```python
from build123d import *
from OCP.BRepFilletAPI import BRepFilletAPI_MakeChamfer

# Parameters (mm, degrees)
SKETCH1_W           = 8
SKETCH1_H           = 19.5
BOSS_EXTRUDE1_DEPTH = 2
FILLET1_R           = 1.6
CUT_EXTRUDE1_DEPTH  = 0.1
SKETCH4_R           = 2.5
SKETCH4_R_2         = 2.25
BOSS_EXTRUDE2_DEPTH = 0.2
CHAMFER1_SIZE       = 0.15
CHAMFER1_SIZE2      = 0.08660254
SKETCH5_W           = 8
SKETCH5_H           = 0.1
CUT_EXTRUDE2_DEPTH  = 1
FILLET2_R           = 0.1


with BuildPart() as part:
    # Sketch1 → Boss-Extrude1 (new body)
    with BuildSketch(Plane.XY):
        with Locations((4, 9.75)):
            Rectangle(SKETCH1_W, SKETCH1_H)
    extrude(amount=BOSS_EXTRUDE1_DEPTH)

    # Fillet1
    fillet1_edges = [part.edges().sort_by_distance(p)[0] for p in [
        (0, 19.5, 1),
        (8, 19.5, 1),
        (8, 0, 1),
        (0, 0, 1),
    ]]
    fillet(fillet1_edges, radius=FILLET1_R)

    # Sketch3 → Cut-Extrude1 (cut)
    with BuildSketch(Plane.XY.offset(2)):
        with BuildLine():
            Line((4.35, 17.3), (4.35, 16.1))
            ThreePointArc((4.35, 16.1), (4, 15.75), (3.65, 16.1))
            Line((3.65, 16.1), (3.65, 17.3))
            ThreePointArc((3.65, 17.3), (4, 17.65), (4.35, 17.3))
        make_face()
        with BuildLine():
            ThreePointArc((2.649265581, 16.627272727), (4, 14.65), (5.350734419, 16.627272727))
            ThreePointArc((5.350734419, 16.627272727), (4.897422349, 16.826039343), (4.698655734, 16.372727273))
            ThreePointArc((4.698655734, 16.372727273), (4, 15.35), (3.301344266, 16.372727273))
            ThreePointArc((3.301344266, 16.372727273), (3.102577651, 16.826039343), (2.649265581, 16.627272727))
        make_face()
    extrude(amount=-CUT_EXTRUDE1_DEPTH, mode=Mode.SUBTRACT)

    # Sketch4 → Boss-Extrude2 (add)
    with BuildSketch(Plane.XY.offset(2)):
        with Locations(Location((4, 16.1, 0), (0, 0, 180))):
            Circle(SKETCH4_R)
        with Locations((4, 16.1)):
            Circle(SKETCH4_R_2, mode=Mode.SUBTRACT)
    extrude(amount=BOSS_EXTRUDE2_DEPTH)

    # Chamfer1: one chamfer whose edges measure the first distance from different faces: ONE call of the kernel's chamfer builder (chamfer() names one face for all edges)
    chamfer1_edges_1 = [part.edges().sort_by_distance(p)[0] for p in [
        (6.5, 16.1, 2.2),
    ]]
    chamfer1_side_1 = [part.faces().sort_by_distance(p)[0] for p in [
        (6.5, 16.1, 2.1),
    ]]
    chamfer1_edges_2 = [part.edges().sort_by_distance(p)[0] for p in [
        (1.75, 16.1, 2.2),
    ]]
    chamfer1_side_2 = [part.faces().sort_by_distance(p)[0] for p in [
        (6.429289322, 16.1, 2.2),
    ]]
    chamfer1 = BRepFilletAPI_MakeChamfer(part.part.solid().wrapped)
    for e in chamfer1_edges_1:
        chamfer1.Add(CHAMFER1_SIZE, CHAMFER1_SIZE2, e.wrapped, chamfer1_side_1[0].wrapped)  # the first distance lies on this face
    for e in chamfer1_edges_2:
        chamfer1.Add(CHAMFER1_SIZE, CHAMFER1_SIZE2, e.wrapped, chamfer1_side_2[0].wrapped)  # the first distance lies on this face
    add(Compound.cast(chamfer1.Shape()), mode=Mode.REPLACE)

    # Sketch5 → Cut-Extrude2 (cut)
    with BuildSketch(Plane.XY.offset(2)):
        with Locations((4, 12.45)):
            Rectangle(SKETCH5_W, SKETCH5_H)
    extrude(amount=-CUT_EXTRUDE2_DEPTH, mode=Mode.SUBTRACT)

    # Fillet2
    # the kernel refuses this fillet: 0.1 mm, written as the material it adds along each edge
    with BuildSketch(Plane(origin=(4, 16.1, 2), x_dir=(-1, 0, 0), z_dir=(0, 1, 0))) as fillet2_piece_1:
        with BuildLine():
            CenterArc((2.58660254, 0.1), FILLET2_R, 210, 60)
            Line((2.58660254, 0), (2.5, 0))
            Line((2.5, 0), (2.5, 0.05))
        make_face()
    revolve(axis=Axis((4, 16.1, 2), (0, 0, 1)))
    # the kernel refuses this fillet: 0.1 mm, written as the material it takes off along each edge
    with BuildSketch(Plane(origin=(8, 1.6, 2), x_dir=(0, 0, -1), z_dir=(0, 1, 0)), Plane(origin=(0, 12.65, 2), x_dir=(0, 0, -1), z_dir=(0, -1, 0))) as fillet2_2_piece_1:
        with BuildLine():
            CenterArc((FILLET2_R, FILLET2_R), FILLET2_R, 180, 90)
            Line((0, FILLET2_R), (0, 0))
            Line((0, 0), (FILLET2_R, 0))
        make_face()
    extrude(amount=11.05, mode=Mode.SUBTRACT)
    with BuildSketch(Plane(origin=(1.6, 0, 2), x_dir=(0, 1, 0), z_dir=(1, 0, 0)), Plane(origin=(6.4, 19.5, 2), x_dir=(0, -1, 0), z_dir=(-1, 0, 0))) as fillet2_2_piece_2:
        with BuildLine():
            CenterArc((FILLET2_R, -FILLET2_R), FILLET2_R, 90, 90)
            Line((0, -FILLET2_R), (0, 0))
            Line((0, 0), (FILLET2_R, 0))
        make_face()
    extrude(amount=4.8, mode=Mode.SUBTRACT)
    with BuildSketch(Plane(origin=(0, 17.9, 2), x_dir=(1, 0, 0), z_dir=(0, -1, 0)), Plane(origin=(8, 12.25, 2), x_dir=(-1, 0, 0), z_dir=(0, 1, 0))) as fillet2_2_piece_3:
        with BuildLine():
            CenterArc((FILLET2_R, -FILLET2_R), FILLET2_R, 90, 90)
            Line((0, -FILLET2_R), (0, 0))
            Line((0, 0), (FILLET2_R, 0))
        make_face()
    extrude(amount=5.65, mode=Mode.SUBTRACT)
    with BuildSketch(Plane(origin=(1.6, 17.9, 2), x_dir=(0, 1, 0), z_dir=(1, 0, 0))) as fillet2_2_piece_4:
        with BuildLine():
            CenterArc((1.6 - FILLET2_R, -FILLET2_R), FILLET2_R, 0, 90)
            Line((1.6, -FILLET2_R), (1.6, 0))
            Line((1.6, 0), (1.6 - FILLET2_R, 0))
        make_face()
    revolve(axis=Axis((1.6, 17.9, 2), (0, 0, 1)), revolution_arc=90, mode=Mode.SUBTRACT)
    with BuildSketch(Plane(origin=(6.4, 17.9, 2), x_dir=(1, 0, 0), z_dir=(0, -1, 0))) as fillet2_2_piece_5:
        with BuildLine():
            CenterArc((1.6 - FILLET2_R, -FILLET2_R), FILLET2_R, 0, 90)
            Line((1.6, -FILLET2_R), (1.6, 0))
            Line((1.6, 0), (1.6 - FILLET2_R, 0))
        make_face()
    revolve(axis=Axis((6.4, 17.9, 2), (0, 0, 1)), revolution_arc=90, mode=Mode.SUBTRACT)
    with BuildSketch(Plane(origin=(1.6, 1.6, 2), x_dir=(0, -1, 0), z_dir=(1, 0, 0))) as fillet2_2_piece_6:
        with BuildLine():
            CenterArc((1.6 - FILLET2_R, FILLET2_R), FILLET2_R, 270, 90)
            Line((1.6 - FILLET2_R, 0), (1.6, 0))
            Line((1.6, 0), (1.6, FILLET2_R))
        make_face()
    revolve(axis=Axis((1.6, 1.6, 2), (0, 0, -1)), revolution_arc=90, mode=Mode.SUBTRACT)
    with BuildSketch(Plane(origin=(6.4, 1.6, 2), x_dir=(0, -1, 0), z_dir=(-1, 0, 0))) as fillet2_2_piece_7:
        with BuildLine():
            CenterArc((1.6 - FILLET2_R, -FILLET2_R), FILLET2_R, 0, 90)
            Line((1.6, -FILLET2_R), (1.6, 0))
            Line((1.6, 0), (1.6 - FILLET2_R, 0))
        make_face()
    revolve(axis=Axis((6.4, 1.6, 2), (0, 0, 1)), revolution_arc=90, mode=Mode.SUBTRACT)
    with BuildSketch(Plane(origin=(8.25, 12.4, 2), x_dir=(0, -1, 0), z_dir=(-1, 0, 0)), Plane(origin=(-0.25, 12.5, 2), x_dir=(0, 1, 0), z_dir=(1, 0, 0))) as fillet2_2_piece_8:
        with BuildLine():
            CenterArc((FILLET2_R, -FILLET2_R), FILLET2_R, 90, 90)
            Line((0, -FILLET2_R), (0, 0))
            Line((0, 0), (FILLET2_R, 0))
        make_face()
    extrude(amount=8.5, mode=Mode.SUBTRACT)


solid = part.part
```
Part model, mm, in its own coordinate system. A direction names the side the tool comes from. Round coordinates to 2 decimals unless told otherwise and drop trailing zeros. Order: outer loops, then holes, each group sorted by start corner. A loop starts at its lowest first (then second) coordinate and runs counter-clockwise, first axis right, second up. Notation, with made-up numbers: M -2,75.25 L 20,75.25 A18 cw 20,90.25 Z; hole C -36,84 d8. An arc over 180 degrees is marked long. Put each result on its own line as item: value. Start each with the question number.
1. Tool access for faces 1 (the face through (0, 10, 1)), 2 (the face through (4.5, 16.1, 2)), 3 (the face through (4, 6, 2)): list every direction of +Z, -Z, +X, -X, +Y, -Y with a clear straight run to the whole face (end or side of a thin tool).
2. Two-plate mould, pull along Y, no slides. Class faces 4 (the face through (0.46, 0.48, 0.96)), 5 (the face through (4, 10, 0)), 6 (the face through (4, 15, 1.9)): +Y half, -Y half, draft (parallel to the pull), parting line (faces both ways), or undercut.
3. Slice it at B-B on y = 9. List the corners of the cut face in (x, z).
4. Drop flat-ended pins along their axis: pin 1 (0.8 mm diameter, centred on x = 4, y = 16.5, fed in from +Z); pin 2 (1 mm diameter, centred on x = 4.5, y = 16, fed in from -Z). Give the stop position or say it passes through.
5. Slice it at A-A on z = 1.65. List the corners of the cut face in (x, y), then the cut area to 3 significant figures.
6. Drill centre lines: probe 1 along Z at (x, y) = (2.5, 8.25); probe 2 along Y at (x, z) = (1.25, 0.75). Where is each one in solid material? Low to high. Write a range as [from, to].
Findings:
1. face 1: +Z, -Z, -X, +Y, -Y
1. face 2: +Z
1. face 3: +Z, +X, -X, -Y
2. face 4: -Y half
2. face 5: draft
2. face 6: undercut
3. outline: M 0,0 L 8,0 L 8,1.9 A0.1 ccw 7.9,2 L 0.1,2 A0.1 ccw 0,1.9 Z
4. pin 1: z = 2
4. pin 2: z = 0
5. outline: M 0,1.6 A1.6 ccw 1.6,0 L 6.4,0 A1.6 ccw 8,1.6 L 8,12.4 L 0,12.4 Z; M 0,12.5 L 8,12.5 L 8,17.9 A1.6 ccw 6.4,19.5 L 1.6,19.5 A1.6 ccw 0,17.9 Z
5. area: 153 mm2
6. probe 1: [0, 2]
6. probe 2: [0.04, 19.46]
